Work out the finished part from the listing and answer in its coordinate system (mm). Face numbers are marked on the shaded views. A direction names the side the tool comes from. Coordinates: 2 decimals unless noted, no trailing zeros. Loops run counter-clockwise (first coordinate to the right, second up) from the corner with the lowest first, then second, coordinate; pieces in that order, holes last. Notation, with made-up numbers: (-34, -21) -> (-18, -21) arc R14 cw to (-18, 3) -> close; hole circle Ø8 at (48, 53). An arc over 180 degrees is marked (long way). Use a Markdown table: item, result.
from build123d import *

# Parameters (mm, degrees)
BOSS_EXTRUDE1_DEPTH = 22.5
SKETCH2_R           = 9.25
SKETCH2_R_2         = 1.7
CUT_EXTRUDE1_DEPTH  = 53.129646076
SKETCH3_R           = 1.7
CUT_EXTRUDE2_DEPTH  = 75.204110398
BOSS_EXTRUDE4_DEPTH = 5
BOSS_EXTRUDE5_DEPTH = 5


with BuildPart() as part:
    # Sketch1 → Boss-Extrude1 (new, symmetric)
    with BuildSketch(Plane(origin=(0, 0, 0), x_dir=(-1, 0, 0), z_dir=(0, 1, 0))):
        Polygon((-33.5, 50), (-16.5, 50), (-16.5, 17), (33.5, 17), (33.5, 0), (-33.5, 0), align=None)
    extrude(amount=BOSS_EXTRUDE1_DEPTH, both=True)

    # Sketch2 → Cut-Extrude1 (cut, through all)
    with BuildSketch(Plane.XY.offset(17)):
        with Locations((-8.5, 0)):
            Circle(SKETCH2_R)
        with Locations((-8.5, 14)):
            Circle(SKETCH2_R_2)
        with Locations((5.5, 0)):
            Circle(SKETCH2_R_2)
        with Locations((-8.5, -14)):
            Circle(SKETCH2_R_2)
        with Locations((-22.5, 0)):
            Circle(SKETCH2_R_2)
    extrude(amount=-CUT_EXTRUDE1_DEPTH, mode=Mode.SUBTRACT)

    # Sketch3 → Cut-Extrude2 (cut, through all)
    with BuildSketch(Plane(origin=(16.5, 0, 0), x_dir=(0, -1, 0), z_dir=(-1, 0, 0))):
        with Locations(Location((12.5, 40, 0), (0, 0, 90))):
            Circle(SKETCH3_R)
        with Locations(Location((-12.5, 40, 0), (0, 0, 90))):
            Circle(SKETCH3_R)
        with Locations(Location((12.5, 27, 0), (0, 0, 270))):
            Circle(SKETCH3_R)
        with Locations(Location((-12.5, 27, 0), (0, 0, 270))):
            Circle(SKETCH3_R)
    extrude(amount=-CUT_EXTRUDE2_DEPTH, mode=Mode.SUBTRACT)

    # Sketch8 → Boss-Extrude4 (add)
    with BuildSketch(Plane(origin=(0, 22.5, 0), x_dir=(-1, 0, 0), z_dir=(0, 1, 0))):
        Polygon((-16.5, 42), (8.5, 17), (-16.5, 17), align=None)
    extrude(amount=-BOSS_EXTRUDE4_DEPTH)

    # Sketch9 → Boss-Extrude5 (add)
    with BuildSketch(Plane.XZ.offset(22.5)):
        Polygon((-8.5, 17), (16.5, 17), (16.5, 42), align=None)
    extrude(amount=-BOSS_EXTRUDE5_DEPTH)


solid = part.part
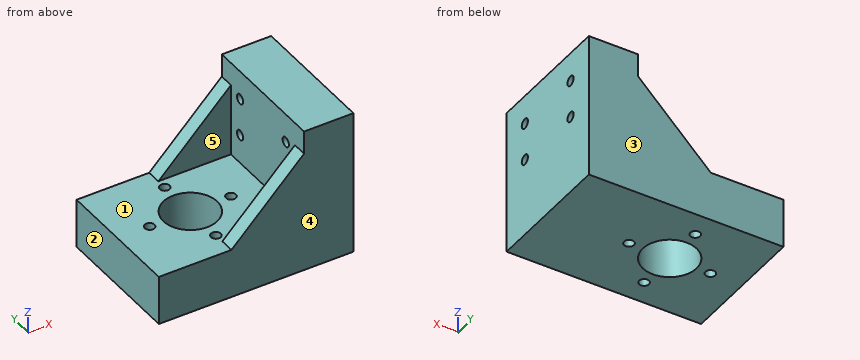
Q1. For the marked faces 4 and 5, determine the directions among +Z, -Z, +X, -X, +Y, -Y from which every point of the face is accessible in a straight line to the end or side of a thin tool.
Solved:
| item | result |
|---|---|
| face 4 | +Z, -Z, +X, -X, -Y |
| face 5 | +Z, -X |
Q2. Section C-C on x = 25.5 is taken. Determine the outline of the cut face in (y, z).
Solved:
| item | result |
|---|---|
| outline | (-22.5, 0) -> (22.5, 0) -> (22.5, 50) -> (-22.5, 50) -> close; hole circle Ø3.4 at (-12.5, 27); hole circle Ø3.4 at (-12.5, 40); hole circle Ø3.4 at (12.5, 27); hole circle Ø3.4 at (12.5, 40) |
Q3. Given pin 1 Ø4 at (x, y) = (-8.5, -14) entering from +Z; pin 2 Ø10 at (x, y) = (2.5, 16) entering from +Z; pin 3 Ø10 at (y, z) = (-6.5, 34) entering from -X, each flat-ended and moving along its own axis, determine where each tip first touches the part or whether it passes through.
Solved:
| item | result |
|---|---|
| pin 1 | z = 17 |
| pin 2 | z = 32.77 |
| pin 3 | x = 16.5 |
Q4. Consider line 1 (Y direction, x = 21.5, z = 27); line 2 (Z direction, x = 24, y = 12); line 3 (Y direction, x = 5.5, z = 6). Determine where each line is inside the solid, lowest interval first. Write a range as [from, to].
Solved:
| item | result |
|---|---|
| line 1 | [-22.5, -14.2], [-10.8, 10.8], [14.2, 22.5] |
| line 2 | [0, 25.38], [28.62, 38.38], [41.62, 50] |
| line 3 | [-22.5, -1.7], [1.7, 22.5] |
Q5. Determine the mould class of the marked faces 1, 2 and 3 for opening direction Y: pulls with the +Y half, pulls with the -Y half, needs draft (parallel to the pull), parting line crosses it, or undercut.
Solved:
| item | result |
|---|---|
| face 1 | undercut |
| face 2 | needs draft |
| face 3 | pulls with the +Y half |
Q6. Section B-B on x = -22.5 is taken. Determine the outline of the cut face in (y, z).
Solved:
| item | result |
|---|---|
| outline | (-22.5, 0) -> (-1.7, 0) -> (-1.7, 17) -> (-22.5, 17) -> close; (1.7, 0) -> (22.5, 0) -> (22.5, 17) -> (1.7, 17) -> close |
Q7. Section D-D on z = 30 is taken. Determine the outline of the cut face in (x, y), and give its area (3 significant figures).
Solved:
| item | result |
|---|---|
| outline | (4.5, -22.5) -> (33.5, -22.5) -> (33.5, 22.5) -> (4.5, 22.5) -> (4.5, 17.5) -> (16.5, 17.5) -> (16.5, -17.5) -> (4.5, -17.5) -> close |
| area | 885 mm² |
Q8. Section A-A on z = 40 is taken. Determine the outline of the cut face in (x, y).
Solved:
| item | result |
|---|---|
| outline | (14.5, -22.5) -> (33.5, -22.5) -> (33.5, -14.2) -> (16.5, -14.2) -> (16.5, -17.5) -> (14.5, -17.5) -> close; (14.5, 17.5) -> (16.5, 17.5) -> (16.5, 14.2) -> (33.5, 14.2) -> (33.5, 22.5) -> (14.5, 22.5) -> close; (16.5, -10.8) -> (33.5, -10.8) -> (33.5, 10.8) -> (16.5, 10.8) -> close |
